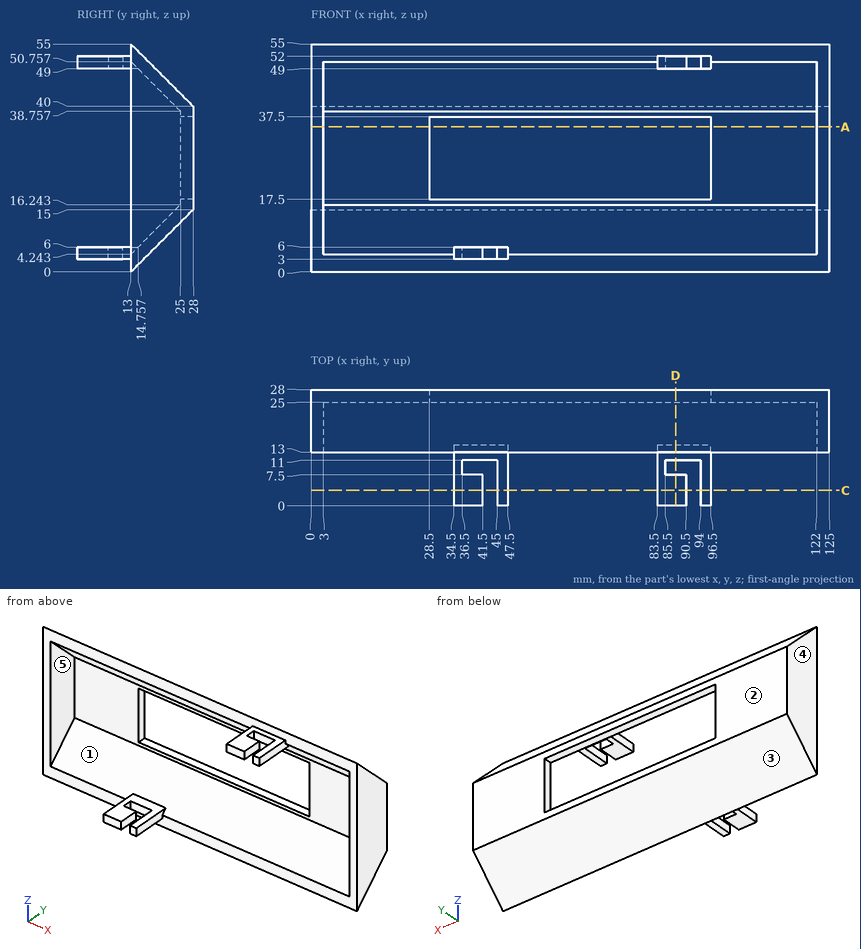
Check sheet for the drawn part. Datum: minimum x, y, z corner. Units: mm. A direction names the side the tool comes from. Give positions to 0.01 mm unless a question says otherwise; leave off trailing zeros. Order: outer loops, then holes, each group sorted by start corner. A loop starts at its lowest first (then second) coordinate and runs counter-clockwise, first axis right, second up. Notation, with made-up numbers: (-25.75, 51) -> (-12.75, 51) arc R29 cw to (-12.75, 90) -> close; hole circle Ø2 at (30, -32). An arc over 180 degrees is marked (long way). One line per item, written item: value.
(1) Tool access check on the marked faces 4 and 5. Record the directions out of +Z, -Z, +X, -X, +Y, -Y that give a thin tool (end or side, any length) a straight path to the whole face; none if there is none.
Final values:
face 4: +Z, -Z, -X, +Y, -Y
face 5: -Y
(2) Scan lines: line 1 along X through (y, z) = (26, 23.5); line 2 along X through (y, z) = (16, 39); line 3 along Y through (x, z) = (21.5, 21.5). Record each from-to range of solid material in increasing order. Write a range as [from, to].
Final values:
line 1: [0, 28.5], [96.5, 125]
line 2: [0, 3], [122, 125]
line 3: [25, 28]
(3) Draft check along Z on the marked faces 1, 2 and 3. Enter one of: pulls with the +Z half, pulls with the -Z half, needs draft (parallel to the pull), parting line crosses it, or undercut.
Final values:
face 1: undercut
face 2: needs draft
face 3: pulls with the -Z half
(4) Sectioned sample at C-C on y = 3.75. Record the cut outline in (x, z), then the cut area to 3 significant figures.
Final values:
outline: (34.5, 3) -> (41.5, 3) -> (41.5, 6) -> (34.5, 6) -> close; (45, 3) -> (47.5, 3) -> (47.5, 6) -> (45, 6) -> close; (83.5, 49) -> (90.5, 49) -> (90.5, 52) -> (83.5, 52) -> close; (94, 49) -> (96.5, 49) -> (96.5, 52) -> (94, 52) -> close
area: 57.0 mm^2
(5) Gauge pin test, flat ends, axial feed: pin 1 (8 mm diameter, centred on x = 95.5, y = 5.5, fed in from -Z); pin 2 (1.5 mm diameter, centred on x = 78.5, y = 26, fed in from +Z); pin 3 (4 mm diameter, centred on x = 110, z = 34.5, fed in from -Y). Record the tip position at first contact, or that the pin passes through.
Final values:
pin 1: z = 49
pin 2: z = 42.75
pin 3: y = 25
(6) Sectioned sample at A-A on z = 35. Record the cut outline in (x, y).
Final values:
outline: (0, 13) -> (3, 13) -> (3, 25) -> (28.5, 25) -> (28.5, 28) -> (0, 28) -> close; (96.5, 25) -> (122, 25) -> (122, 13) -> (125, 13) -> (125, 28) -> (96.5, 28) -> close
(7) Sectioned sample at D-D on x = 88. Count the separate pieces of the cut face and the enclosed holes in it, then the cut area to 3 significant figures.
Final values:
separate pieces: 3
enclosed holes: 0
area: 156 mm^2
